Job drawing, mm, ordinate dimensions from the low corner. One solid piece. A direction names the side the tool comes from. Coordinates: 2 decimals unless noted, no trailing zeros. Order: outer loops, then holes, each group sorted by start corner. A loop starts at its lowest first (then second) coordinate and runs counter-clockwise, first axis right, second up. Notation, with made-up numbers: (-25.75, 50) - (-0.75, 50) arc R8 cw to (-0.75, 61) - close; hole circle Ø1 at (32.25, 70.25). An arc over 180 degrees is marked (long way). Use a Markdown table: item, result. Add a question column.
1) Wall check: L1, parallel to Y at x = 112, z = 41 (1 decimal). Give the ranges that are in metal, low to high. Write a range as [from, to].
2) Saw through at C-C on x = 82.5. List the corners of the cut face in (y, z) (1 decimal).
3) Two-plate mould, pull along X, no slides. Class the marked faces 3, 4, 5 and 6: +X half, -X half, draft (parallel to the pull), parting line (faces both ways), or undercut.
4) Tool access for the marked faces 1 and 2: list every direction of +Z, -Z, +X, -X, +Y, -Y with a clear straight run to the whole face (end or side of a thin tool).
5) Drop flat-ended pins along their axis: P1, Ø3, axis at y = 128.82, z = 9.95, coming from the -X side; P2, Ø8, axis at x = 128, y = 110, coming from the +Z side (3 decimals); P3, Ø24, axis at x = 100.5, z = 22.5, coming from the +Y side (3 decimals); P4, Ø1, axis at x = 49, z = 2, coming from the +Y side (3 decimals). Give the stop position or say it passes through.
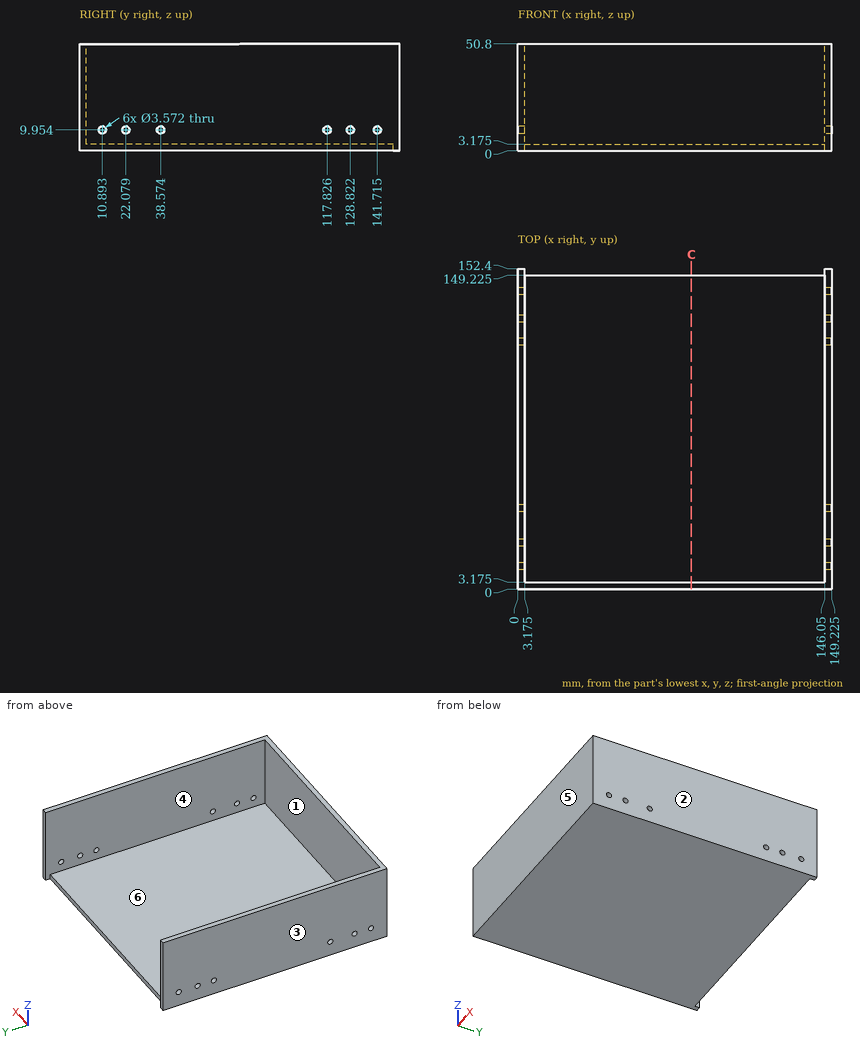
Results are:
| question | item | result |
|---|---|---|
| 1 | L1 | [0, 3.2] |
| 2 | outline | (0, 0) - (149.2, 0) - (149.2, 3.2) - (3.2, 3.2) - (3.2, 50.8) - (0, 50.8) - close |
| 3 | face 3 | -X half |
| 3 | face 4 | undercut |
| 3 | face 5 | draft |
| 3 | face 6 | undercut |
| 4 | face 1 | +Z, +Y |
| 4 | face 2 | +Z, -Z, +X, +Y, -Y |
| 5 | P1 | through |
| 5 | P2 | z = 3.175 |
| 5 | P3 | y = 3.175 |
| 5 | P4 | y = 149.225 |
